Build history of the part. All positions in model axes, mm. Coordinates: 2 decimals unless noted, no trailing zeros. Loops run counter-clockwise (first coordinate to the right, second up) from the corner with the lowest first, then second, coordinate; pieces in that order, holes last.
(1) Slice it at D-D (z = -4.75). Give the cut face in (x, y) (3 decimals), and give its area (3 significant figures).
(2) Slice it at C-C (y = 0). Give the cut face in (x, z), and give its area (3 significant figures).
(3) Two-plate mould, pull along Z, no slides. Class faces 1 (the face through (42.884, 0.608, -9.534)), 2 (the face through (-42.884, 0.608, -9.534)), 3 (the face through (-49.8, 0, -9)), 4 (the face through (0, 6, -3)): pulls with the +Z half, pulls with the -Z half, needs draft (parallel to the pull), parting line crosses it, or undercut.
(4) Slice it at A-A (x = 0). Give the cut face in (y, z), and give its area (3 significant figures).
(5) Wall check: L1, parallel to Y at x = 43, z = -11; L2, parallel to X at y = -2.5, z = -10.5; L3, parallel to Z at x = -20.5, y = 13. Give the ranges that are in metal, low to high.
(6) Slice it at B-B (z = -11). Give the cut face in (x, y), and give its area (3 significant figures).
(7) Flat gauge pins, fed straight in: P1, Ø16, axis at x = 0, y = 0, coming from the -Z side; P2, Ø3, axis at y = 0, z = -11, coming from the -X side; P3, Ø1, axis at x = -32.5, y = 12.5, coming from the +Z side; P4, Ø12, axis at x = 9.5, y = 10.5, coming from the +Z side. Where does each tip first touch, or does it go through?
from build123d import *

# Parameters (mm, degrees)
SKETCH5_W                         = 25
SKETCH5_H                         = 25
CUT_EXTRUDE3_DEPTH                = 1
F_1_8_0_125_DIAMETER_HOLE2_REACH  = 115.234
F_1_8_0_125_DIAMETER_HOLE2_BORE_R = 1.5875


with BuildPart() as part:
    # Sketch2 → Revolve1 (revolve)
    with BuildSketch(Plane(origin=(0, 0, 0), x_dir=(0, 0, -1), z_dir=(1, 0, 0)), mode=Mode.PRIVATE) as revolve1_sk:
        Polygon((0, 30), (7, 50.8), (15, 50.8), (15, 40.8), (3, 30), (3, 5), (0, 5), align=None)
    revolve(revolve1_sk.sketch.rotate(Axis((0, 0, 1000), (0, 0, -1)), 90), axis=Axis((0, 0, 1000), (0, 0, -1)))

    # Sketch5 → Cut-Extrude3 (cut)
    with BuildSketch(Plane(origin=(50.8, 0, 0), x_dir=(0, 0, -1), z_dir=(1, 0, 0))):
        with Locations((10, 0)):
            Rectangle(SKETCH5_W, SKETCH5_H)
    cut_extrude3 = extrude(amount=-CUT_EXTRUDE3_DEPTH, mode=Mode.SUBTRACT)

    # 1/8 (0.125) Diameter Hole2 bore (on position points) → 1/8 (0.125) Diameter Hole2 (cut, up to next)
    with BuildSketch(Plane(origin=(49.8, 0, -11), x_dir=(0, 0, 1), z_dir=(1, 0, 0)), mode=Mode.PRIVATE) as f_1_8_0_125_diameter_hole2_sk1:
        Circle(F_1_8_0_125_DIAMETER_HOLE2_BORE_R)
    f_1_8_0_125_diameter_hole2_tool1 = extrude(f_1_8_0_125_diameter_hole2_sk1.sketch, amount=-F_1_8_0_125_DIAMETER_HOLE2_REACH, mode=Mode.PRIVATE) & part.part
    f_1_8_0_125_diameter_hole2 = f_1_8_0_125_diameter_hole2_tool1.solids().sort_by_distance((49.8, 0, -11))[0]
    add(f_1_8_0_125_diameter_hole2, mode=Mode.SUBTRACT)

    # Mirror2: Cut-Extrude3, 1/8 (0.125) Diameter Hole2 across plane
    add(cut_extrude3.mirror(Plane(origin=(0, 0, 0), x_dir=(0, 0, 1), z_dir=(1, 0, 0))), mode=Mode.SUBTRACT)
    add(f_1_8_0_125_diameter_hole2.mirror(Plane(origin=(0, 0, 0), x_dir=(0, 0, 1), z_dir=(1, 0, 0))), mode=Mode.SUBTRACT)


solid = part.part
Response values:
1. outline: circle Ø88.229 at (0, 0); hole circle Ø63.15 at (0, 0)
1. area: 2,980 mm2
2. outline: (-49.8, -15) - (-40.8, -15) - (-38.63, -12.59) - (-49.8, -12.59) - close; (-49.8, -9.41) - (-35.77, -9.41) - (-30, -3) - (-5, -3) - (-5, 0) - (-30, 0) - (-49.8, -6.66) - close; (5, -3) - (30, -3) - (35.77, -9.41) - (49.8, -9.41) - (49.8, -6.66) - (30, 0) - (5, 0) - close; (38.63, -12.59) - (40.8, -15) - (49.8, -15) - (49.8, -12.59) - close
2. area: 402 mm2
3. face 1: undercut
3. face 2: undercut
3. face 3: needs draft
3. face 4: pulls with the -Z half
4. outline: (-50.8, -15) - (-40.8, -15) - (-30, -3) - (-5, -3) - (-5, 0) - (-30, 0) - (-50.8, -7) - close; (5, -3) - (30, -3) - (40.8, -15) - (50.8, -15) - (50.8, -7) - (30, 0) - (5, 0) - close
4. area: 499 mm2
5. L1: y = -27.05 to -1.59, 1.59 to 27.05
5. L2: x = -49.8 to -36.66, 36.66 to 49.8
5. L3: z = -3 to 0
6. outline: (-49.8, -10.03) arc R50.8 ccw to (49.8, -10.03) - (49.8, -1.59) - (37.17, -1.59) arc R37.2 cw to (-37.17, -1.59) - (-49.8, -1.59) - close; (-49.8, 1.59) - (-37.17, 1.59) arc R37.2 cw to (37.17, 1.59) - (49.8, 1.59) - (49.8, 10.03) arc R50.8 ccw to (-49.8, 10.03) - close
6. area: 3,650 mm2
7. P1: stops at z = -3
7. P2: passes through
7. P3: stops at z = -1.45
7. P4: stops at z = 0
